```python
from build123d import *
from build123d.topology import SkipClean

# Parameters (mm, degrees)
SKETCH1_R               = 1.6
SKETCH1_R_2             = 1
SKETCH1_R_3             = 5.5
SKETCH1_R_4             = 4.5
BOSS_EXTRUDE2_DEPTH     = 2
BOSS_EXTRUDE3_START     = -2
SKETCH2_R               = 1
BOSS_EXTRUDE3_DEPTH     = 2
SKETCH3_R               = 1
CUT_EXTRUDE1_DEPTH      = 103
BOSS_EXTRUDE4_OUTLINE_R = 1
BOSS_EXTRUDE4_DEPTH     = 10
SKETCH5_R               = 87.063932705
CUT_EXTRUDE2_DEPTH      = 2
BOSS_EXTRUDE5_START     = 2
SKETCH6_R               = 1
SKETCH6_R_2             = 1.6
SKETCH6_R_3             = 4.5
BOSS_EXTRUDE5_DEPTH     = 2
SKETCH7_R               = 66.92041454
CUT_EXTRUDE3_DEPTH      = 10
SKETCH8_R               = 1.6
CUT_EXTRUDE4_DEPTH      = 10
BOSS_EXTRUDE6_DEPTH     = 2


# Read off the part's stored shape, not the designer's step: Boss-Extrude4
with BuildPart() as part:
    # Sketch1 → Boss-Extrude2 (new body)
    with BuildSketch(Plane(origin=(0, 0, 0), x_dir=(1, 0, 0), z_dir=(0, 1, 0))):
        with BuildLine():
            Line((12.313589515, -16.493996637), (35.979225245, -12.848450001))
            ThreePointArc((35.979225245, -12.848450001), (46.993067566, -0.424494085), (36.813648041, 12.691862933))
            Line((36.813648041, 12.691862933), (35.165189196, 12.947676785))
            Line((35.165189196, 12.947676785), (12.319067304, 16.493021261))
            ThreePointArc((12.319067304, 16.493021261), (11.720527595, 16.549330191), (11.119556233, 16.533395936))
            Line((11.119556233, 16.533395936), (-11.812019178, 14.541098507))
            ThreePointArc((-11.812019178, 14.541098507), (-13.247239988, 14.027709898), (-14.244912332, 12.87528787))
            Line((-14.244912332, 12.87528787), (-19.487592157, 2.204884721))
            ThreePointArc((-19.487592157, 2.204884721), (-19.693653105, -1.723258696), (-16.994761113, -4.584858569))
            Line((-16.994761113, -4.584858569), (9.557587922, -16.137143667))
            ThreePointArc((9.557587922, -16.137143667), (10.910298182, -16.51089082), (12.313589515, -16.493996637))
        make_face()
        with Locations(Location((11.552349036, -11.552285098, 0), (0, 0, 270))):
            Circle(SKETCH1_R, mode=Mode.SUBTRACT)
        with Locations(Location((25, -11, 0), (0, 0, 270))):
            Circle(SKETCH1_R_2, mode=Mode.SUBTRACT)
        with Locations(Location((-15, 0, 0), (0, 0, 270))):
            Circle(SKETCH1_R, mode=Mode.SUBTRACT)
        with Locations(Location((0, 0, 0), (0, 0, 270))):
            Circle(SKETCH1_R_3, mode=Mode.SUBTRACT)
        with Locations(Location((-11.552357038, 11.552357038, 0), (0, 0, 270))):
            Circle(SKETCH1_R, mode=Mode.SUBTRACT)
        with Locations(Location((11.552326466, 11.552160153, 0), (0, 0, 270))):
            Circle(SKETCH1_R, mode=Mode.SUBTRACT)
        with Locations(Location((14, 0, 0), (0, 0, 270))):
            Circle(SKETCH1_R_4, mode=Mode.SUBTRACT)
        with Locations(Location((34, 0, 0), (0, 0, 270))):
            Circle(SKETCH1_R_4, mode=Mode.SUBTRACT)
        with Locations(Location((25, 11, 0), (0, 0, 270))):
            Circle(SKETCH1_R_2, mode=Mode.SUBTRACT)
    extrude(amount=BOSS_EXTRUDE2_DEPTH)

    # Sketch2 → Boss-Extrude3 (add)
    with BuildSketch(Plane(origin=(0, 2, 0), x_dir=(1, 0, 0), z_dir=(0, 1, 0)).offset(BOSS_EXTRUDE3_START)):
        with Locations((25, 11)):
            Circle(SKETCH2_R)
        with Locations((25, -11)):
            Circle(SKETCH2_R)
    extrude(amount=BOSS_EXTRUDE3_DEPTH)

    # Sketch3 → Cut-Extrude1 (cut)
    with BuildSketch(Plane(origin=(0, 2, 0), x_dir=(1, 0, 0), z_dir=(0, 1, 0))):
        with Locations(Location((24, 13, 0), (0, 0, 270))):
            Circle(SKETCH3_R)
        with Locations(Location((24, -13, 0), (0, 0, 270))):
            Circle(SKETCH3_R)
    extrude(amount=-CUT_EXTRUDE1_DEPTH, mode=Mode.SUBTRACT)

    # Boss-Extrude4 outline → Boss-Extrude4 (add)
    with SkipClean():  # the faces are left unmerged after this step: merging them gives an invalid solid
        with BuildSketch(Plane(origin=(0, 2, 0), x_dir=(1, 0, 0), z_dir=(0, 1, 0))):
            with BuildLine():
                ThreePointArc((8.453372169, -15.47610242), (10.277484332, -16.387026041), (12.313589515, -16.493996637))
                Line((12.313589515, -16.493996637), (35.979225245, -12.848450001))
                ThreePointArc((35.979225245, -12.848450001), (46.993067566, -0.424494085), (36.813648041, 12.691862933))
                Line((36.813648041, 12.691862933), (12.319067304, 16.493021261))
                ThreePointArc((12.319067304, 16.493021261), (10.294223964, 16.391290043), (8.476229775, 15.493940099))
                Line((8.476229775, 15.493940099), (-4.306535369, 5.518491924))
                ThreePointArc((-4.306535369, 5.518491924), (-7, 0), (-4.306535369, -5.518491924))
                Line((-4.306535369, -5.518491924), (8.453372169, -15.47610242))
            make_face()
            with Locations((24, -13)):
                Circle(BOSS_EXTRUDE4_OUTLINE_R, mode=Mode.SUBTRACT)
            with BuildLine():
                Line((35.738243971, -12.126046672), (26.117255626, -13.608064851))
                Line((26.117255626, -13.608064851), (25.976685738, -12.695511096))
                ThreePointArc((25.976685738, -12.695511096), (23.695511096, -11.023314262), (22.023314262, -13.304488904))
                Line((22.023314262, -13.304488904), (22.16388415, -14.217042659))
                Line((22.16388415, -14.217042659), (12.27862862, -15.739768587))
                ThreePointArc((12.27862862, -15.739768587), (10.519552717, -15.67488522), (8.937649363, -14.902784407))
                Line((8.937649363, -14.902784407), (-3.845146577, -4.927204867))
                ThreePointArc((-3.845146577, -4.927204867), (-6.249813783, 0.048245957), (-3.768620923, 4.985979978))
                Line((-3.768620923, 4.985979978), (9.140409076, 14.743187339))
                ThreePointArc((9.140409076, 14.743187339), (10.553310252, 15.425397379), (12.119916334, 15.511685597))
                Line((12.119916334, 15.511685597), (22.133828609, 14.076211769))
                Line((22.133828609, 14.076211769), (22.020237278, 13.283794934))
                ThreePointArc((22.020237278, 13.283794934), (23.716205066, 11.020237278), (25.979762722, 12.716205066))
                Line((25.979762722, 12.716205066), (26.093354053, 13.508621901))
                Line((26.093354053, 13.508621901), (35.738243971, 12.126046672))
                ThreePointArc((35.738243971, 12.126046672), (46.25, 0), (35.738243971, -12.126046672))
            make_face(mode=Mode.SUBTRACT)
            with Locations((24, 13)):
                Circle(BOSS_EXTRUDE4_OUTLINE_R, mode=Mode.SUBTRACT)
        extrude(amount=BOSS_EXTRUDE4_DEPTH)
    add(part.part.scale(1), mode=Mode.REPLACE)  # the faces are merged on a copy

    # Sketch5 → Cut-Extrude2 (cut)
    with BuildSketch(Plane(origin=(0, 0, 0), x_dir=(-1, 0, 0), z_dir=(0, -1, 0))):
        Circle(SKETCH5_R)
    extrude(amount=-CUT_EXTRUDE2_DEPTH, mode=Mode.SUBTRACT)

    # Sketch6 → Boss-Extrude5 (add)
    with BuildSketch(Plane(origin=(0, 2, 0), x_dir=(-1, 0, 0), z_dir=(0, -1, 0)).offset(BOSS_EXTRUDE5_START)):
        with BuildLine():
            Line((4.306535369, -5.518491924), (-8.453372169, -15.47610242))
            ThreePointArc((-8.453372169, -15.47610242), (-10.277484331, -16.387026041), (-12.313589515, -16.493996637))
            Line((-12.313589515, -16.493996637), (-35.979225245, -12.848450001))
            ThreePointArc((-35.979225245, -12.848450001), (-46.993067566, -0.424494085), (-36.813648041, 12.691862933))
            Line((-36.813648041, 12.691862933), (-12.319067304, 16.493021261))
            ThreePointArc((-12.319067304, 16.493021261), (-10.294223964, 16.391290043), (-8.476229775, 15.493940099))
            Line((-8.476229775, 15.493940099), (4.306535369, 5.518491924))
            ThreePointArc((4.306535369, 5.518491924), (7, 0), (4.306535369, -5.518491924))
        make_face()
        with Locations(Location((-24, -13, 0), (0, 0, 270))):
            Circle(SKETCH6_R, mode=Mode.SUBTRACT)
        with Locations(Location((-24, 13, 0), (0, 0, 270))):
            Circle(SKETCH6_R, mode=Mode.SUBTRACT)
        with Locations(Location((0, 0, 0), (0, 0, 90))):
            Circle(SKETCH6_R_2, mode=Mode.SUBTRACT)
        with Locations(Location((-34, 0, 0), (0, 0, 90))):
            Circle(SKETCH6_R_3, mode=Mode.SUBTRACT)
        with Locations(Location((-14, 0, 0), (0, 0, 90))):
            Circle(SKETCH6_R_3, mode=Mode.SUBTRACT)
    extrude(amount=-BOSS_EXTRUDE5_DEPTH)

    # Sketch7 → Cut-Extrude3 (cut)
    with BuildSketch(Plane(origin=(0, 12, 0), x_dir=(1, 0, 0), z_dir=(0, 1, 0))):
        Circle(SKETCH7_R)
    extrude(amount=-CUT_EXTRUDE3_DEPTH, mode=Mode.SUBTRACT)

    # Sketch8 → Cut-Extrude4 (cut)
    with BuildSketch(Plane(origin=(0, 0, 0), x_dir=(-1, 0, 0), z_dir=(0, -1, 0))):
        with Locations((-24, -12.25)):
            Circle(SKETCH8_R)
        with Locations((-24, 12.25)):
            Circle(SKETCH8_R)
    extrude(amount=-CUT_EXTRUDE4_DEPTH, mode=Mode.SUBTRACT)

    # Sketch9 → Boss-Extrude6 (add)
    with BuildSketch(Plane(origin=(0, 0, 0), x_dir=(-1, 0, 0), z_dir=(0, -1, 0))):
        with BuildLine():
            ThreePointArc((-24.746843357, -13.665), (-24, -13.85), (-23.253156643, -13.665))
            ThreePointArc((-23.253156643, -13.665), (-24, -14), (-24.746843357, -13.665))
        make_face()
        with BuildLine():
            ThreePointArc((-23.253156643, 13.665), (-24, 13.85), (-24.746843357, 13.665))
            ThreePointArc((-24.746843357, 13.665), (-24, 14), (-23.253156643, 13.665))
        make_face()
    extrude(amount=-BOSS_EXTRUDE6_DEPTH)


solid = part.part
```
The listing builds one solid part. Answer for the finished solid, in the listing's coordinates (mm). Coordinates: 2 decimals unless noted, no trailing zeros. Order: outer loops, then holes, each group sorted by start corner. A loop starts at its lowest first (then second) coordinate and runs counter-clockwise, first axis right, second up. Notation, with made-up numbers: M 49,47 L 76,47 A25 ccw 76,60 Z; hole C 63,5.5 d11. An arc over 180 degrees is marked long. Answer as a JSON object with one key per item and string values. Group by question number.
1. Section C-C on x = 0 is taken. Write down the section's boundary in (y, z).
2. Section D-D on z = 12.25 is taken. Write down the section's boundary in (x, y), then the cut area to 3 significant figures.
3. Section A-A on z = 0 is taken. Write down the section's boundary in (x, y), then the cut area to 3 significant figures.
4. Straight lines are drawn through the part: line 1 (X direction, y = 1.1, z = 0); line 2 (Z direction, x = 23.5, y = 0.95); line 3 (X direction, y = 0.5, z = -3). For each, find the intervals that lie inside material, in ascending order.
5. Determine the mould class of faces 1 (the cylindrical face through (29.61, 0.99, 0.98)), 2 (the flat face through (1.984, 0.986, 10.428)), 3 (the cylindrical face through (-7, 1, 0)) for opening direction Z: released by +Z, released by -Z, zero draft, split by the parting line, or undercut.
6. Section B-B on y = 0.9 is taken. State how many separate pieces and enclosed holes the cut face has, then the cut area to 3 significant figures.
Values follow:
{
 "1": {"outline": "M 0,-8.88 L 2,-8.88 L 2,-1.6 L 0,-1.6 Z; M 0,1.6 L 2,1.6 L 2,8.88 L 0,8.88 Z"},
 "2": {"outline": "M 4.32,0 L 22.4,0 L 22.4,2 L 4.32,2 Z; M 25.6,0 L 38.35,0 L 38.35,2 L 25.6,2 Z", "area": "61.7 mm2"},
 "3": {"outline": "M -7,0 L -1.6,0 L -1.6,2 L -7,2 Z; M 1.6,0 L 9.5,0 L 9.5,2 L 1.6,2 Z; M 18.5,0 L 29.5,0 L 29.5,2 L 18.5,2 Z; M 38.5,0 L 47,0 L 47,2 L 38.5,2 Z", "area": "65.6 mm2"},
 "4": {"line 1": "-7 to -1.6, 1.6 to 9.5, 18.5 to 29.5, 38.5 to 47", "line 2": "-14.76 to -13.77, -10.73 to 10.73, 13.77 to 14.77", "line 3": "-6.32 to 10.65, 17.35 to 30.65, 37.35 to 46.65"},
 "5": {"face 1": "undercut", "face 2": "released by +Z", "face 3": "split by the parting line"},
 "6": {"separate pieces": "1", "enclosed holes": "5", "area": "1,170 mm2"}
}
